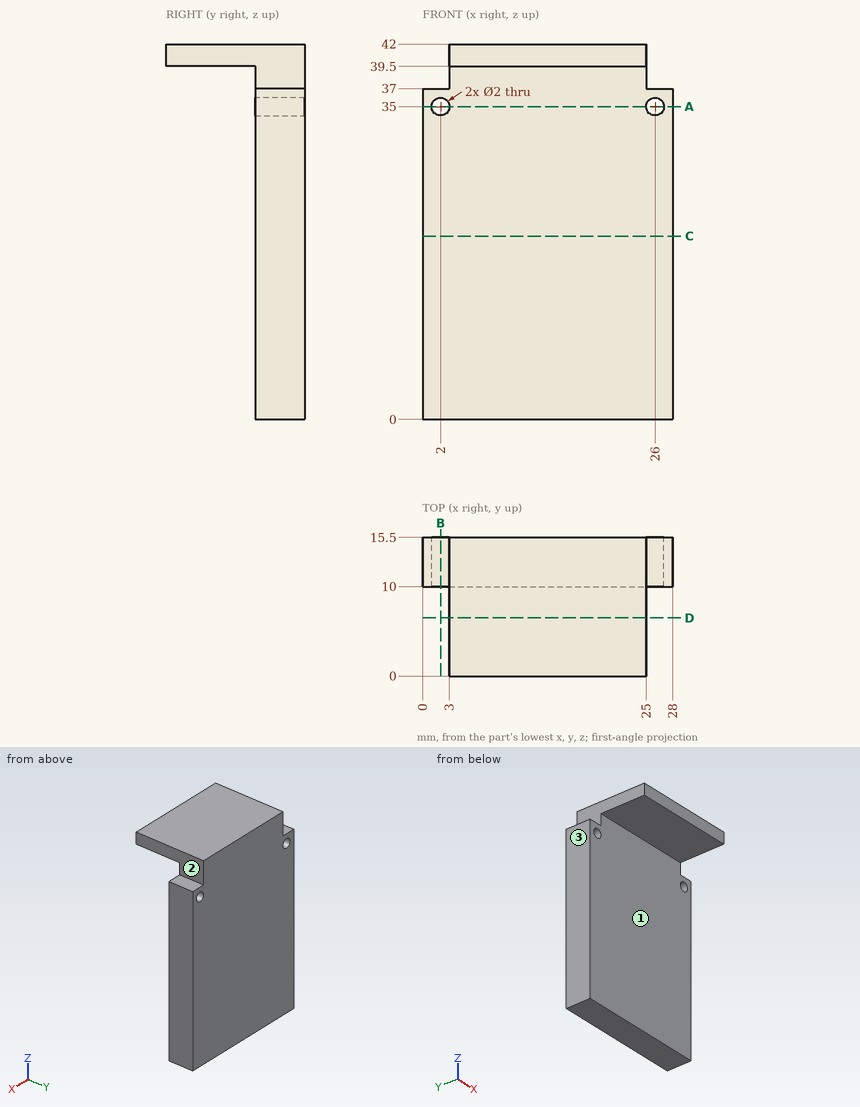
The drawing under review shows one solid part. Ordinate dimensions are in mm from its lowest x, y, z. A direction names the side the tool comes from. Coordinates: 2 decimals unless noted, no trailing zeros. Write each loop counter-clockwise with the first axis right and the second up, starting at its lowest first coordinate (ties: lowest second). Pieces come first, ordered by that corner, then holes. Notation, with made-up numbers: M -14.5,70 L -8.5,70 A27 ccw -8.5,93 Z; hole C 47,69 d1. An arc over 180 degrees is marked long. Put each result on its own line as item: value.
1) Add section A-A on z = 35. Give the boundary of the cut face in (x, y), then the cut area to 3 significant figures.
Computed:
outline: M 0,10 L 1,10 L 1,15.5 L 0,15.5 Z; M 3,10 L 25,10 L 25,15.5 L 3,15.5 Z; M 27,10 L 28,10 L 28,15.5 L 27,15.5 Z
area: 132 mm2
2) Add section C-C on z = 20.5. Give the boundary of the cut face in (x, y), then the cut area to 3 significant figures.
Computed:
outline: M 0,10 L 28,10 L 28,15.5 L 0,15.5 Z
area: 154 mm2
3) Wall thickness on probe 1 along X at (y, z) = (11.7, 35); probe 2 along Y at (x, z) = (2.5, 24); probe 3 along Z at (x, y) = (7, 9.5): over which ranges is each line inside the solid? List them lowest first. Write a range as [from, to].
Computed:
probe 1: x = [0, 1], [3, 25], [27, 28]
probe 2: y = [10, 15.5]
probe 3: z = [39.5, 42]
4) Add section D-D on y = 6.5. Give the boundary of the cut face in (x, z), then the cut area to 3 significant figures.
Computed:
outline: M 3,39.5 L 25,39.5 L 25,42 L 3,42 Z
area: 55.0 mm2
5) Clearance check with flat-ended pins moving along their axes: pin 1 Ø4 at (x, z) = (5, 4.5) entering from -Y; pin 2 Ø8 at (y, z) = (3.5, 5) entering from -X; pin 3 Ø2.5 at (x, y) = (27, 13) entering from +Z; pin 4 Ø1.5 at (y, z) = (6.5, 40.5) entering from -X. State where each tip first meets the part, or that it passes through.
Computed:
pin 1: stops at y = 10
pin 2: passes through
pin 3: stops at z = 37
pin 4: stops at x = 3
6) For the marked faces 1, 2 and 3, list the 3-axis set-ups (+Z, -Z, +X, -X, +Y, -Y) from which the entire face can be reached by the end or side of a thin tool; tool diameter is ignored.
Computed:
face 1: -Z, +X, -X, -Y
face 2: +Z, +X, +Y, -Y
face 3: +Z, -Z, -X, +Y, -Y
7) Add section B-B on x = 2. Give the boundary of the cut face in (y, z), then the cut area to 4 significant figures.
Computed:
outline: M 10,0 L 15.5,0 L 15.5,34 L 10,34 Z; M 10,36 L 15.5,36 L 15.5,37 L 10,37 Z
area: 192.5 mm2
